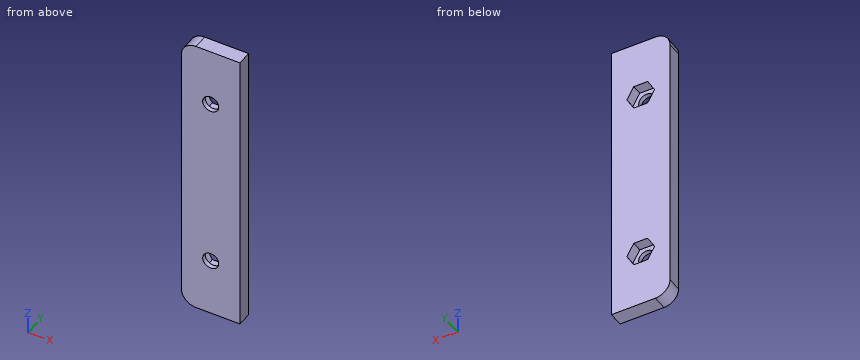
Autodesk Inventor part; units mm, degrees
ref_plane "YZ Plane" through (0, 0, 0) normal (1, 0, 0) x (0, 1, 0)
ref_plane "XZ Plane" through (0, 0, 0) normal (0, 1, 0) x (-1, 0, 0)
ref_plane "XY Plane" through (0, 0, 0) normal (0, 0, 1) x (1, 0, 0)
sketch "Sketch1" plane through (0, 0, 0) normal (0, 1, 0) x (-1, 0, 0)
  line L0 (-10, 50) -> (10, 50)
  line L1 (10, 50) -> (10, -50)
  line L2 (10, -50) -> (-10, -50)
  line L3 (-10, -50) -> (-10, 50)
  line L4 (-10, 50) -> (10, -50) construction
  line L5 (10, 50) -> (-10, -50) construction
  circle A0 centre (0, 30) radius 2.75
  circle A1 centre (0, -30) radius 2.75
  point P0 (0, 0)
  dimension "d0" = 20
  dimension "d1" = 100
  dimension "d2" = 5.5
  dimension "d3" = 20
  dimension "d4" = 20
extrude "Extrusion1" add sketch "Sketch1" along normal blind 5
sketch "Sketch2" plane through (0, 5, 0) normal (0, 1, 0) x (1, 0, 0)
  circle A0 centre (0, -30) radius 2.75
  circle A1 centre (0, -30) radius 4.1
  circle A2 centre (0, 30) radius 2.75
  circle A3 centre (0, 30) radius 4.1
  line L0 (-4.7343, -30) -> (-2.3671, -25.9)
  line L1 (-2.3671, -25.9) -> (2.3671, -25.9)
  line L2 (2.3671, -25.9) -> (4.7343, -30)
  line L3 (4.7343, -30) -> (2.3671, -34.1)
  line L4 (2.3671, -34.1) -> (-2.3671, -34.1)
  line L5 (-2.3671, -34.1) -> (-4.7343, -30)
  line L6 (-4.7343, 30) -> (-2.3671, 34.1)
  line L7 (-2.3671, 34.1) -> (2.3671, 34.1)
  line L8 (2.3671, 34.1) -> (4.7343, 30)
  line L9 (4.7343, 30) -> (2.3671, 25.9)
  line L10 (2.3671, 25.9) -> (-2.3671, 25.9)
  line L11 (-2.3671, 25.9) -> (-4.7343, 30)
  point P0 (0, 0)
  dimension "d7" = 8.2
extrude "Extrusion2" cut sketch "Sketch2" against normal blind 3.5 contours A0 | A1 | A1 L2 L3 | A1 L1 L2 | L3 L4 A1 | A1 L0 L1 | L4 L5 A1 | A1 L5 L0 | A2 | A3 | A3 L8 L9 | A3 L7 L8 | L9 L10 A3 | A3 L6 L7 | L10 L11 A3 | A3 L11 L6
fillet "Fillet1" radius 5 2 edges at (-10, 2.5, 50) (-10, 2.5, -50)
properties part number "Rubberplate"
Verification items for the finished model (mm, model axes). Give positions to 0.01 mm unless a question says otherwise; leave off trailing zeros. Order: outer loops, then holes, each group sorted by start corner. A loop starts at its lowest first (then second) coordinate and runs counter-clockwise, first axis right, second up. Notation, with made-up numbers: M 21,48 L 67,48 A3 ccw 67,52 Z; hole C 88.25,72.5 d4. An arc over 180 degrees is marked long. Answer in a Markdown table with one row per item. Add a question column.
Item 1: Scan lines: probe 1 along Z at (x, y) = (0, 0.95); probe 2 along Z at (x, y) = (2, 4.5); probe 3 along X at (y, z) = (0.8, -30). Record each from-to range of solid material in increasing order. Write a range as from..to.
Item 2: Section check C-C, the plane z = 31. Enter the section's corners in (x, y), and give its area (3 significant figures).
Item 3: Section check B-B, the plane x = 0.5. Enter the section's corners in (y, z).
Item 4: Section check A-A, the plane y = 4.1. Enter the section's corners in (x, z), and give its area (3 significant figures).
Item 5: Gauge pin test, flat ends, axial feed: pin 1 (9 mm diameter, centred on x = -2.5, z = -29, fed in from +Y); pin 2 (7 mm diameter, centred on x = 0, z = 30, fed in from +Y). Record the tip position at first contact, or that the pin passes through.
Filled sheet:
| question | item | result |
|---|---|---|
| 1 | probe 1 | z = -50..-32.75, -27.25..27.25, 32.75..50 |
| 1 | probe 2 | z = -50..-34.1, -25.9..25.9, 34.1..50 |
| 1 | probe 3 | x = -10..-2.75, 2.75..10 |
| 2 | outline | M -10,0 L -2.56,0 L -2.56,1.5 L -4.16,1.5 L -4.16,5 L -10,5 Z; M 2.56,0 L 10,0 L 10,5 L 4.16,5 L 4.16,1.5 L 2.56,1.5 Z |
| 2 | area | 63.2 mm^2 |
| 3 | outline | M 0,-50 L 5,-50 L 5,-34.1 L 1.5,-34.1 L 1.5,-32.7 L 0,-32.7 Z; M 0,-27.3 L 1.5,-27.3 L 1.5,-25.9 L 5,-25.9 L 5,25.9 L 1.5,25.9 L 1.5,27.3 L 0,27.3 Z; M 0,32.7 L 1.5,32.7 L 1.5,34.1 L 5,34.1 L 5,50 L 0,50 Z |
| 4 | outline | M -10,-45 A5 ccw -5,-50 L 10,-50 L 10,50 L -5,50 A5 ccw -10,45 Z; hole M -4.73,-30 L -2.37,-34.1 L 2.37,-34.1 L 4.73,-30 L 2.37,-25.9 L -2.37,-25.9 Z; hole M -4.73,30 L -2.37,25.9 L 2.37,25.9 L 4.73,30 L 2.37,34.1 L -2.37,34.1 Z |
| 4 | area | 1,870 mm^2 |
| 5 | pin 1 | stops at y = 5 |
| 5 | pin 2 | stops at y = 1.5 |
